from build123d import *

# Parameters (mm, degrees)
BOSS_EXTRUDE1_START       = -2
SKETCH2_W                 = 74.7
SKETCH2_H                 = 59.6
BOSS_EXTRUDE1_DEPTH       = 2
BOSS_EXTRUDE2_START       = -2
SKETCH3_W                 = 74.7
SKETCH3_H                 = 59.6
SKETCH3_W_2               = 70.7
SKETCH3_H_2               = 55.6
BOSS_EXTRUDE2_DEPTH       = 3.5
BOSS_EXTRUDE3_START       = -4
SKETCH4_R                 = 2.5
BOSS_EXTRUDE3_DEPTH       = 4
M3X0_5_TAPPED_HOLE2_D     = 2.5
M3X0_5_TAPPED_HOLE2_DEPTH = 2.5
M3X0_5_TAPPED_HOLE2_TIP   = 0.751075774
FILLET1_R                 = 0.75
FILLET2_R                 = 2
SKETCH15_W                = 2
SKETCH15_H                = 13
SKETCH15_H_2              = 16.1
CUT_EXTRUDE1_DEPTH        = 0.5


with BuildPart() as part:
    # Sketch2 → Boss-Extrude1 (new body)
    with BuildSketch(Plane(origin=(0, 0, 0), x_dir=(1, 0, 0), z_dir=(0, 1, 0)).offset(BOSS_EXTRUDE1_START)):
        with Locations((34.35, 26.8)):
            Rectangle(SKETCH2_W, SKETCH2_H)
    extrude(amount=-BOSS_EXTRUDE1_DEPTH)

    # Sketch3 → Boss-Extrude2 (add)
    with BuildSketch(Plane(origin=(0, 0, 0), x_dir=(1, 0, 0), z_dir=(0, 1, 0)).offset(BOSS_EXTRUDE2_START)):
        with Locations((34.35, 26.8)):
            Rectangle(SKETCH3_W, SKETCH3_H)
        with Locations((34.35, 26.8)):
            Rectangle(SKETCH3_W_2, SKETCH3_H_2, mode=Mode.SUBTRACT)
    extrude(amount=BOSS_EXTRUDE2_DEPTH)

    # Sketch4 → Boss-Extrude3 (add)
    with BuildSketch(Plane(origin=(0, 0, 0), x_dir=(1, 0, 0), z_dir=(0, 1, 0)).offset(BOSS_EXTRUDE3_START)):
        with Locations(Location((14, 2.5, 0), (0, 0, 270))):
            Circle(SKETCH4_R)
        with Locations(Location((15, 51.1, 0), (0, 0, 270))):
            Circle(SKETCH4_R)
        with Locations(Location((66.2, 33.5, 0), (0, 0, 270))):
            Circle(SKETCH4_R)
        with Locations(Location((66, 7.5, 0), (0, 0, 270))):
            Circle(SKETCH4_R)
    extrude(amount=BOSS_EXTRUDE3_DEPTH)

    # M3x0.5 Tapped Hole2
    with Locations(Plane(origin=(66, 0, -7.5), x_dir=(0, 0, 1), z_dir=(0, 1, 0))):
        with Locations((0, 0), (-26, 0.2), (-43.6, -51), (5, -52)):
            Hole(M3X0_5_TAPPED_HOLE2_D / 2, depth=M3X0_5_TAPPED_HOLE2_DEPTH)
            with Locations((0, 0, -(M3X0_5_TAPPED_HOLE2_DEPTH + M3X0_5_TAPPED_HOLE2_TIP / 2))):  # 118° drill point
                Cone(0, M3X0_5_TAPPED_HOLE2_D / 2, M3X0_5_TAPPED_HOLE2_TIP, mode=Mode.SUBTRACT)

    # Fillet1
    fillet1_edges = [part.edges().sort_by_distance(p)[0] for p in [
        (-1, -0.25, 1),
        (-1, -0.25, -54.6),
        (69.7, -0.25, -54.6),
        (69.7, -0.25, 1),
    ]]
    fillet(fillet1_edges, radius=FILLET1_R)

    # Fillet2
    fillet2_edges = [part.edges().sort_by_distance(p)[0] for p in [
        (71.7, -1.25, -56.6),
        (71.7, -1.25, 3),
        (-3, -1.25, 3),
        (-3, -1.25, -56.6),
    ]]
    fillet(fillet2_edges, radius=FILLET2_R)

    # Sketch15 → Cut-Extrude1 (cut)
    with BuildSketch(Plane(origin=(0, 1.5, 0), x_dir=(1, 0, 0), z_dir=(0, 1, 0))):
        with Locations((-2, 8.75)):
            Rectangle(SKETCH15_W, SKETCH15_H)
        with Locations((-2, 39.05)):
            Rectangle(SKETCH15_W, SKETCH15_H_2)
    extrude(amount=-CUT_EXTRUDE1_DEPTH, mode=Mode.SUBTRACT)


solid = part.part
Read the model definition and answer for the solid it produces. Units are mm, in the model's axes. A direction names the side the tool comes from. Give positions to 0.01 mm unless a question says otherwise; leave off trailing zeros. Loops run counter-clockwise (first coordinate to the right, second up) from the corner with the lowest first, then second, coordinate; pieces in that order, holes last. Notation, with made-up numbers: (50.25, 50) -> (58.25, 50) arc R31 ccw to (58.25, 83) -> close; hole circle Ø3 at (65.5, 53.25). An arc over 180 degrees is marked (long way). Use a Markdown table: item, result.
Q1. Each of these flat-tipped pins is pushed along its axis until it touches: pin 1 (2 mm diameter, centred on x = -2, z = -41, fed in from +Y); pin 2 (1.5 mm diameter, centred on x = 66.5, z = -34, fed in from +Y); pin 3 (0.6 mm diameter, centred on x = -2, y = 1, fed in from +Z). Where does it stop, or does it pass through?
Solved:
| item | result |
|---|---|
| pin 1 | stops at y = 1 |
| pin 2 | stops at y = 0 |
| pin 3 | stops at z = 2.87 |
Q2. A tool of negligible diameter and unlimited length cuts with its end or side. For faces 5 (the face through (34, -1, -56.6)), 6 (the face through (34, 0, -54.6)), 7 (the face through (-2, 1, -39)), from which of +Z, -Z, +X, -X, +Y, -Y can it reach the whole face along a straight path? Write none if from no direction.
Solved:
| item | result |
|---|---|
| face 5 | -Z, +X, -X, +Y, -Y |
| face 6 | +Y |
| face 7 | -X, +Y |
Q3. Find the intervals of material crossed by line 1 along X through (y, z) = (-1.9, -33.5); line 2 along X through (y, z) = (-0.5, -7.5); line 3 along Z through (x, y) = (17, 0.9), in increasing order.
Solved:
| item | result |
|---|---|
| line 1 | x = -3 to -1, 63.7 to 64.95, 67.45 to 68.7, 69.7 to 71.7 |
| line 2 | x = -3 to -1, 63.5 to 64.75, 67.25 to 68.5, 69.7 to 71.7 |
| line 3 | z = -56.6 to -54.6, 1 to 3 |
Q4. Determine the mould class of faces 1 (the face through (70, 1.5, -27)), 2 (the face through (68.48, -1.01, -7.83)), 3 (the face through (13, 0, -4)), 4 (the face through (-2.43, -1.29, -56)) for opening direction Z: pulls with the +Z half, pulls with the -Z half, needs draft (parallel to the pull), parting line crosses it, or undercut.
Solved:
| item | result |
|---|---|
| face 1 | needs draft |
| face 2 | undercut |
| face 3 | undercut |
| face 4 | pulls with the -Z half |
Q5. Section B-B, the plane z = -44.5 is taken. Determine the outline of the cut face in (x, y).
Solved:
| item | result |
|---|---|
| outline | (-3, -4) -> (71.7, -4) -> (71.7, 1.5) -> (69.7, 1.5) -> (69.7, -2) -> (-1, -2) -> (-1, 1) -> (-3, 1) -> close |
Q6. Section A-A, the plane x = 30.5 is taken. Determine the outline of the cut face in (y, z).
Solved:
| item | result |
|---|---|
| outline | (-4, -56.6) -> (1.5, -56.6) -> (1.5, -54.6) -> (-2, -54.6) -> (-2, 1) -> (1.5, 1) -> (1.5, 3) -> (-4, 3) -> close |
